Geometry: final body of the model. Coordinates: model frame, mm. Give positions to 0.01 mm unless a question says otherwise; leave off trailing zeros. Loops run counter-clockwise (first coordinate to the right, second up) from the corner with the lowest first, then second, coordinate; pieces in that order, holes last. Notation, with made-up numbers: (58, 50) - (63, 50) arc R16 ccw to (63, 75) - close; hole circle Ø2 at (-34, -20.75). An arc over 180 degrees is marked (long way). Answer in a Markdown table with one row per item.
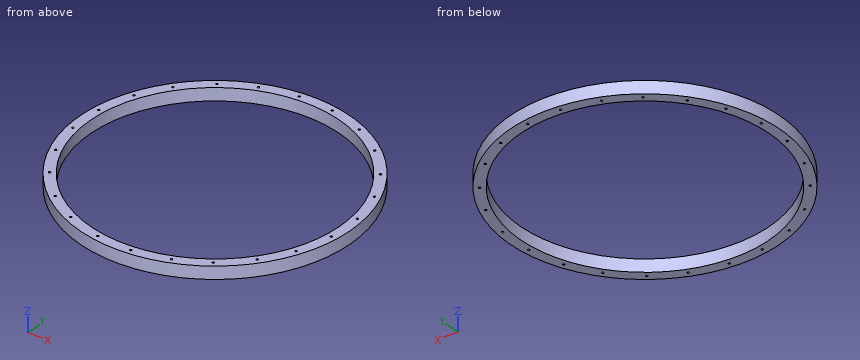
from build123d import *

# Parameters (mm, degrees)
F0_R     = 130
F0_R_2   = 120
F1_DEPTH = 12


with BuildPart() as f1:
    # F0 (on Top) → F1 (new body)
    with BuildSketch(Plane.XY):
        Circle(F0_R)
        with BuildLine():
            ThreePointArc((115.533661, -47.045387), (116.153821, -47.377912), (116.401407, -48.036603))
            ThreePointArc((116.401407, -48.036603), (115.729346, -48.981302), (114.616495, -48.65621))
            Line((114.616495, -48.65621), (99.915499, -74.475656))
            ThreePointArc((99.915499, -74.475656), (100.285226, -74.84207), (100.420705, -75.344666))
            ThreePointArc((100.420705, -75.344666), (99.806158, -76.267393), (98.717854, -76.056003))
            Line((98.717854, -76.056003), (76.532392, -98.509331))
            ThreePointArc((76.532392, -98.509331), (76.819507, -98.860115), (76.922249, -99.301622))
            ThreePointArc((76.922249, -99.301622), (75.994508, -100.299008), (74.932692, -99.445762))
            Line((74.932692, -99.445762), (49.291532, -114.45556))
            ThreePointArc((49.291532, -114.45556), (49.393668, -114.699031), (49.428523, -114.960747))
            ThreePointArc((49.428523, -114.960747), (48.562023, -115.951796), (47.464168, -115.225358))
            Line((47.464168, -115.225358), (17.02433, -123.577779))
            ThreePointArc((17.02433, -123.577779), (17.08074, -123.764616), (17.099785, -123.958852))
            ThreePointArc((17.099785, -123.958852), (15.911439, -124.940954), (15.170734, -123.588902))
            Line((15.170734, -123.588902), (-14.54006, -123.767188))
            ThreePointArc((-14.54006, -123.767188), (-14.540047, -123.770189), (-14.540042, -123.773189))
            ThreePointArc((-14.540042, -123.773189), (-15.667593, -124.765021), (-16.507504, -123.520171))
            Line((-16.507504, -123.520171), (-47.045387, -115.533661))
            ThreePointArc((-47.045387, -115.533661), (-48.531397, -116.270417), (-48.65621, -114.616495))
            Line((-48.65621, -114.616495), (-74.475656, -99.915499))
            ThreePointArc((-74.475656, -99.915499), (-75.948656, -100.217697), (-76.056003, -98.717854))
            Line((-76.056003, -98.717854), (-98.509331, -76.532392))
            ThreePointArc((-98.509331, -76.532392), (-100.164631, -76.427437), (-99.445762, -74.932692))
            Line((-99.445762, -74.932692), (-114.45556, -49.291532))
            ThreePointArc((-114.45556, -49.291532), (-115.882314, -48.816743), (-115.225358, -47.464168))
            Line((-115.225358, -47.464168), (-123.577779, -17.02433))
            ThreePointArc((-123.577779, -17.02433), (-124.958834, -16.105786), (-123.588902, -15.170734))
            Line((-123.588902, -15.170734), (-123.767188, 14.54006))
            ThreePointArc((-123.767188, 14.54006), (-124.765399, 15.664617), (-123.520171, 16.507504))
            Line((-123.520171, 16.507504), (-115.533661, 47.045387))
            ThreePointArc((-115.533661, 47.045387), (-116.270417, 48.531397), (-114.616495, 48.65621))
            Line((-114.616495, 48.65621), (-99.915499, 74.475656))
            ThreePointArc((-99.915499, 74.475656), (-100.217697, 75.948656), (-98.717854, 76.056003))
            Line((-98.717854, 76.056003), (-76.532392, 98.509331))
            ThreePointArc((-76.532392, 98.509331), (-76.427437, 100.164631), (-74.932692, 99.445762))
            Line((-74.932692, 99.445762), (-49.291532, 114.45556))
            ThreePointArc((-49.291532, 114.45556), (-48.816743, 115.882314), (-47.464168, 115.225358))
            Line((-47.464168, 115.225358), (-17.02433, 123.577779))
            ThreePointArc((-17.02433, 123.577779), (-16.294021, 124.939807), (-15.099785, 123.958852))
            ThreePointArc((-15.099785, 123.958852), (-15.117683, 123.770506), (-15.170734, 123.588902))
            Line((-15.170734, 123.588902), (14.54006, 123.767188))
            ThreePointArc((14.54006, 123.767188), (15.537042, 124.773185), (16.540042, 123.773189))
            ThreePointArc((16.540042, 123.773189), (16.531874, 123.645638), (16.507504, 123.520171))
            Line((16.507504, 123.520171), (47.045387, 115.533661))
            ThreePointArc((47.045387, 115.533661), (48.102875, 116.399209), (49.036603, 115.401407))
            ThreePointArc((49.036603, 115.401407), (48.936494, 114.965292), (48.65621, 114.616495))
            Line((48.65621, 114.616495), (74.475656, 99.915499))
            ThreePointArc((74.475656, 99.915499), (75.600586, 100.387403), (76.344666, 99.420705))
            ThreePointArc((76.344666, 99.420705), (76.26969, 99.040795), (76.056003, 98.717854))
            Line((76.056003, 98.717854), (98.509331, 76.532392))
            ThreePointArc((98.509331, 76.532392), (99.623886, 76.868899), (100.301622, 75.922249))
            ThreePointArc((100.301622, 75.922249), (100.057975, 75.268085), (99.445762, 74.932692))
            Line((99.445762, 74.932692), (114.45556, 49.291532))
            ThreePointArc((114.45556, 49.291532), (115.458147, 49.296045), (115.960747, 48.428523))
            ThreePointArc((115.960747, 48.428523), (115.755923, 47.822145), (115.225358, 47.464168))
            Line((115.225358, 47.464168), (123.577779, 17.02433))
            ThreePointArc((123.577779, 17.02433), (124.515146, 16.93077), (124.958852, 16.099785))
            ThreePointArc((124.958852, 16.099785), (124.520123, 15.272153), (123.588902, 15.170734))
            Line((123.588902, 15.170734), (123.767188, -14.54006))
            ThreePointArc((123.767188, -14.54006), (124.478171, -14.830817), (124.773189, -15.540042))
            ThreePointArc((124.773189, -15.540042), (124.384328, -16.331566), (123.520171, -16.507504))
            Line((123.520171, -16.507504), (115.533661, -47.045387))
        make_face(mode=Mode.SUBTRACT)
        with BuildLine():
            ThreePointArc((114.616495, -48.65621), (114.532397, -47.541809), (115.533661, -47.045387))
            Line((115.533661, -47.045387), (123.520171, -16.507504))
            ThreePointArc((123.520171, -16.507504), (122.780979, -15.415468), (123.767188, -14.54006))
            Line((123.767188, -14.54006), (123.588902, 15.170734))
            ThreePointArc((123.588902, 15.170734), (122.95887, 16.093785), (123.577779, 17.02433))
            Line((123.577779, 17.02433), (115.225358, 47.464168))
            ThreePointArc((115.225358, 47.464168), (114.039181, 48.040303), (114.45556, 49.291532))
            Line((114.45556, 49.291532), (99.445762, 74.932692))
            ThreePointArc((99.445762, 74.932692), (98.438612, 75.417061), (98.509331, 76.532392))
            Line((98.509331, 76.532392), (76.056003, 98.717854))
            ThreePointArc((76.056003, 98.717854), (74.740676, 98.623713), (74.475656, 99.915499))
            Line((74.475656, 99.915499), (48.65621, 114.616495))
            ThreePointArc((48.65621, 114.616495), (47.541809, 114.532397), (47.045387, 115.533661))
            Line((47.045387, 115.533661), (16.507504, 123.520171))
            ThreePointArc((16.507504, 123.520171), (15.415468, 122.780979), (14.54006, 123.767188))
            Line((14.54006, 123.767188), (-15.170734, 123.588902))
            ThreePointArc((-15.170734, 123.588902), (-16.093785, 122.95887), (-17.02433, 123.577779))
            Line((-17.02433, 123.577779), (-47.464168, 115.225358))
            ThreePointArc((-47.464168, 115.225358), (-47.437474, 115.094247), (-47.428523, 114.960747))
            ThreePointArc((-47.428523, 114.960747), (-48.166807, 113.995602), (-49.291532, 114.45556))
            Line((-49.291532, 114.45556), (-74.932692, 99.445762))
            ThreePointArc((-74.932692, 99.445762), (-74.924863, 99.373881), (-74.922249, 99.301622))
            ThreePointArc((-74.922249, 99.301622), (-75.480742, 98.404364), (-76.532392, 98.509331))
            Line((-76.532392, 98.509331), (-98.717854, 76.056003))
            ThreePointArc((-98.717854, 76.056003), (-98.497978, 75.73012), (-98.420705, 75.344666))
            ThreePointArc((-98.420705, 75.344666), (-98.918109, 74.480145), (-99.915499, 74.475656))
            Line((-99.915499, 74.475656), (-114.616495, 48.65621))
            ThreePointArc((-114.616495, 48.65621), (-114.456708, 48.364542), (-114.401407, 48.036603))
            ThreePointArc((-114.401407, 48.036603), (-114.742717, 47.284189), (-115.533661, 47.045387))
            Line((-115.533661, 47.045387), (-123.520171, 16.507504))
            ThreePointArc((-123.520171, 16.507504), (-122.981666, 16.151181), (-122.773189, 15.540042))
            ThreePointArc((-122.773189, 15.540042), (-123.063964, 14.83506), (-123.767188, 14.54006))
            Line((-123.767188, 14.54006), (-123.588902, -15.170734))
            ThreePointArc((-123.588902, -15.170734), (-123.13122, -15.538514), (-122.958852, -16.099785))
            ThreePointArc((-122.958852, -16.099785), (-123.127866, -16.65608), (-123.577779, -17.02433))
            Line((-123.577779, -17.02433), (-115.225358, -47.464168))
            ThreePointArc((-115.225358, -47.464168), (-114.354369, -47.633347), (-113.960747, -48.428523))
            ThreePointArc((-113.960747, -48.428523), (-114.093226, -48.925922), (-114.45556, -49.291532))
            Line((-114.45556, -49.291532), (-99.445762, -74.932692))
            ThreePointArc((-99.445762, -74.932692), (-98.647458, -75.165896), (-98.301622, -75.922249))
            ThreePointArc((-98.301622, -75.922249), (-98.354972, -76.244513), (-98.509331, -76.532392))
            Line((-98.509331, -76.532392), (-76.056003, -98.717854))
            ThreePointArc((-76.056003, -98.717854), (-74.964756, -98.495681), (-74.344666, -99.420705))
            ThreePointArc((-74.344666, -99.420705), (-74.377968, -99.676625), (-74.475656, -99.915499))
            Line((-74.475656, -99.915499), (-48.65621, -114.616495))
            ThreePointArc((-48.65621, -114.616495), (-47.600488, -114.501516), (-47.036603, -115.401407))
            ThreePointArc((-47.036603, -115.401407), (-47.038801, -115.46768), (-47.045387, -115.533661))
            Line((-47.045387, -115.533661), (-16.507504, -123.520171))
            ThreePointArc((-16.507504, -123.520171), (-15.415468, -122.780979), (-14.54006, -123.767188))
            Line((-14.54006, -123.767188), (15.170734, -123.588902))
            ThreePointArc((15.170734, -123.588902), (16.093785, -122.95887), (17.02433, -123.577779))
            Line((17.02433, -123.577779), (47.464168, -115.225358))
            ThreePointArc((47.464168, -115.225358), (48.040303, -114.039181), (49.291532, -114.45556))
            Line((49.291532, -114.45556), (74.932692, -99.445762))
            ThreePointArc((74.932692, -99.445762), (75.417061, -98.438612), (76.532392, -98.509331))
            Line((76.532392, -98.509331), (98.717854, -76.056003))
            ThreePointArc((98.717854, -76.056003), (98.623713, -74.740676), (99.915499, -74.475656))
            Line((99.915499, -74.475656), (114.616495, -48.65621))
        make_face()
        Circle(F0_R_2, mode=Mode.SUBTRACT)
    extrude(amount=F1_DEPTH)


solid = f1.part
Q1. First-contact query: pin 1 (2.5 mm diameter, centred on x = -123.96, y = -16.1, fed in from -Z); pin 2 (4 mm diameter, centred on y = -74, z = 8.5, fed in from +X); pin 3 (3 mm diameter, centred on y = 49.5, z = 6.5, fed in from +X); pin 4 (1.8 mm diameter, centred on x = 16.1, y = -123.96, fed in from -Z). Flat tips, straight axial feed; report the tip coordinate or a pass-through.
Check values:
| item | result |
|---|---|
| pin 1 | z = 0 |
| pin 2 | x = 108.24 |
| pin 3 | x = 120.81 |
| pin 4 | through |
Q2. Cut plane A-A (x = 0). Output: boundary loops of the cut face in (y, z), and give its area (3 significant figures).
Check values:
| item | result |
|---|---|
| outline | (-130, 0) - (-120, 0) - (-120, 12) - (-130, 12) - close; (120, 0) - (130, 0) - (130, 12) - (120, 12) - close |
| area | 240 mm² |
Q3. Material intervals for line 1 along Y through (x, z) = (0, 9.5); line 2 along X through (y, z) = (15, 2.5); line 3 along X through (y, z) = (-44, 7.5), sorted ascending.
Check values:
| item | result |
|---|---|
| line 1 | -130 to -120, 120 to 130 |
| line 2 | -129.13 to -124.61, -122.93 to -119.06, 119.06 to 129.13 |
| line 3 | -122.33 to -111.64, 111.64 to 122.33 |
Q4. Cut plane C-C (z = 9). Give the number of separate pieces and of enclosed holes in the cut face, and give its area (3 significant figures).
Check values:
| item | result |
|---|---|
| separate pieces | 1 |
| enclosed holes | 25 |
| area | 7,780 mm² |
